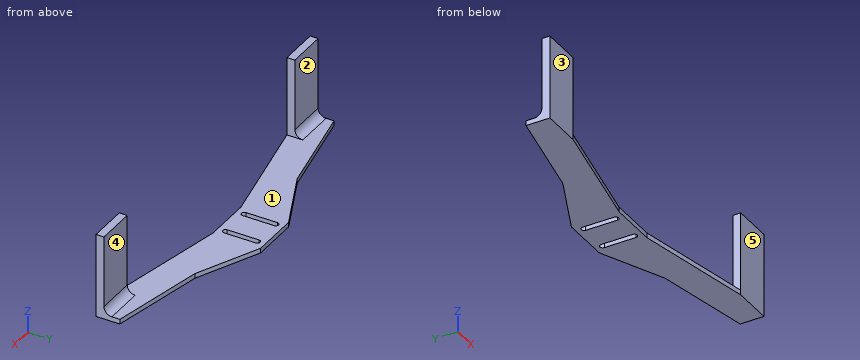
```python
from build123d import *

# Parameters (mm, degrees)
SKETCH_1_W      = 30
SKETCH_1_H      = 30
EXTRUDE_1_DEPTH = 3
EXTRUDE_START   = -3
SKETCH_2_W      = 25
SKETCH_2_H      = 5
EXTRUDE_2_DEPTH = 50
FILLET_1_R      = 5


with BuildPart() as part:
    # 草图1 → 凸台-拉伸1 (new body)
    # profile 1 of 3: a face of its own
    with BuildSketch(Plane.XY):
        Polygon((15, 15), (15, -15), (90, -30), (115, -30), (115, -15), (55, -3), align=None)
    # profile 2 of 3: a face of its own
    with BuildSketch(Plane.XY):
        Rectangle(SKETCH_1_W, SKETCH_1_H)
        with BuildLine():
            Line((-11.75, -10), (-11.75, 10))
            ThreePointArc((-11.75, 10), (-10, 11.75), (-8.25, 10))
            Line((-8.25, 10), (-8.25, -10))
            ThreePointArc((-8.25, -10), (-10, -11.75), (-11.75, -10))
        make_face(mode=Mode.SUBTRACT)
        with BuildLine():
            ThreePointArc((8.25, 10), (10, 11.75), (11.75, 10))
            Line((11.75, 10), (11.75, -10))
            ThreePointArc((11.75, -10), (10, -11.75), (8.25, -10))
            Line((8.25, -10), (8.25, 10))
        make_face(mode=Mode.SUBTRACT)
    # profile 3 of 3: a face of its own
    with BuildSketch(Plane.XY):
        Polygon((-55, -3), (-15, 15), (-15, -15), (-90, -30), (-115, -30), (-115, -15), align=None)
    extrude(amount=EXTRUDE_1_DEPTH)

    # 草图2 → 凸台-拉伸2 (add)
    with BuildSketch(Plane(origin=(0, 0, 0), x_dir=(-1, 0, 0), z_dir=(0, 0, -1)).offset(EXTRUDE_START)):
        with Locations((-102.5, -27.5)):
            Rectangle(SKETCH_2_W, SKETCH_2_H)
        with Locations((102.5, -27.5)):
            Rectangle(SKETCH_2_W, SKETCH_2_H)
    extrude(amount=-EXTRUDE_2_DEPTH)

    # 圆角1
    fillet_1_edges = [part.edges().sort_by_distance(p)[0] for p in [
        (102.5, -25, 3),
        (-102.5, -25, 3),
    ]]
    fillet(fillet_1_edges, radius=FILLET_1_R)


solid = part.part
```
Geometry check sheet. Reference: the model listing, model coordinates, mm. Face numbers are marked on the shaded views. A direction names the side the tool comes from. Give positions to 0.01 mm unless a question says otherwise; leave off trailing zeros. Write each loop counter-clockwise with the first axis right and the second up, starting at its lowest first coordinate (ties: lowest second). Pieces come first, ordered by that corner, then holes. Notation, with made-up numbers: (82.5, 74.25) -> (132.5, 74.25) arc R23 cw to (132.5, 111.25) -> close; hole circle Ø4 at (-2.75, -15.5). An arc over 180 degrees is marked (long way). Use one line per item in the form item = value.
Item 1: Mould release check, pull along Y, two halves, no side actions. Record for the marked faces 1, 2 and 3: released by +Y, released by -Y, zero draft, split by the parting line, or undercut.
Results list:
face_1 = zero draft
face_2 = released by +Y
face_3 = released by -Y
Item 2: Sectioned sample at A-A on y = -5. Enter the section's corners in (x, z), plus the area to 3 significant figures.
Results list:
outline = (-65, 0) -> (-11.75, 0) -> (-11.75, 3) -> (-65, 3) -> close; (-8.25, 0) -> (8.25, 0) -> (8.25, 3) -> (-8.25, 3) -> close; (11.75, 0) -> (65, 0) -> (65, 3) -> (11.75, 3) -> close
area = 369 mm2
Item 3: Sectioned sample at C-C on x = -40. Enter the section's corners in (y, z), plus the area to 4 significant figures.
Results list:
outline = (-20, 0) -> (3.75, 0) -> (3.75, 3) -> (-20, 3) -> close
area = 71.25 mm2
Item 4: Scan lines: line 1 (Z direction, x = 24.5, y = 2); line 2 (Y direction, x = 96, z = 43). Record each from-to range of solid material in increasing order.
Results list:
line_1 = 0 to 3
line_2 = -30 to -25
Item 5: Sectioned sample at B-B on z = 18. Enter the section's corners in (x, y), plus the area to 3 significant figures.
Results list:
outline = (-115, -30) -> (-90, -30) -> (-90, -25) -> (-115, -25) -> close; (90, -30) -> (115, -30) -> (115, -25) -> (90, -25) -> close
area = 250 mm2
Item 6: Depth check by flat-ended pin: pin 1 Ø3.5 at (y, z) = (1.5, 1.5) entering from +X; pin 2 Ø5 at (x, y) = (-28.5, 7) entering from +Z; pin 3 Ø7.5 at (x, z) = (-102, 20.5) entering from +Y. Enter the tip coordinate at first touch or a pass-through.
Results list:
pin_1 = 48.89
pin_2 = 3
pin_3 = -25
Item 7: Sectioned sample at D-D on x = 82. Enter the section's corners in (y, z), plus the area to 3 significant figures.
Results list:
outline = (-28.4, 0) -> (-8.4, 0) -> (-8.4, 3) -> (-28.4, 3) -> close
area = 60.0 mm2
Item 8: Access from +Z, -Z, +X, -X, +Y, -Y to the whole of each face (thin tool, end or side, straight path). Record for the marked faces 4 and 5.
Results list:
face_4 = +Z, +X, -X, +Y
face_5 = +Z, -Z, +X, -X, -Y
